Input: part model. Units: mm. Frame: model coordinates. Round coordinates to 2 decimals unless told otherwise and drop trailing zeros. Loops run counter-clockwise (first coordinate to the right, second up) from the corner with the lowest first, then second, coordinate; pieces in that order, holes last. Notation, with made-up numbers: (30.5, 13.5) - (75.5, 13.5) arc R5 cw to (75.5, 19.5) - close; hole circle Ø8 at (53, 24). An arc over 180 degrees is marked (long way). One line per question, with ' | ' between items. Start each with the question number.
Item 1: Section C-C, the plane z = -57. Return loops of the section in (x, y).
Item 2: Section B-B, the plane y = 1.5. Give the number of separate pieces and of enclosed holes in the cut face, plus the area to 3 significant figures.
Item 3: Section D-D, the plane x = -14. Return loops of the section in (y, z).
Item 4: First-contact query: pin 1 (0.6 mm diameter, centred on y = 1.5, z = -15.5, fed in from +X); pin 2 (12 mm diameter, centred on x = -7.5, z = -46.5, fed in from +Y). Flat tips, straight axial feed; report the tip coordinate or a pass-through.
Item 5: Material intervals for line 1 along Z through (x, y) = (-30, 1.25); line 2 along X through (y, z) = (1.2, -56); line 3 along Z through (x, y) = (-21.5, 0.7), sorted ascending.
Item 6: Section A-A, the plane x = -26. Return loops of the section in (y, z), plus the area to 3 significant figures.
Autodesk Inventor part; units mm, degrees
ref_plane "YZ Plane" through (0, 0, 0) normal (1, 0, 0) x (0, 1, 0)
ref_plane "XZ Plane" through (0, 0, 0) normal (0, 1, 0) x (-1, 0, 0)
ref_plane "XY Plane" through (0, 0, 0) normal (0, 0, 1) x (1, 0, 0)
sketch "Sketch1" plane through (0, 0, 0) normal (0, 1, 0) x (-1, 0, 0)
  line L0 (0, 0) -> (0, -30)
  line L1 (0, 0) -> (0.75, 0) construction
  arc A0 (1.4548, 0.2565) -> (0, 0) centre (0.75, 0) ccw
  line L2 (1.4548, 0.2565) -> (6.5322, -13.6936)
  line L3 (0, -30) -> (0.75, -30) construction
  circle A1 centre (0.75, -30) radius 0.75
  line L4 (1.0065, -30.7048) -> (6.5322, -28.6936)
  line L5 (6.5322, -13.6936) -> (6.5322, -28.6936) construction
  line L6 (6.5322, -13.6936) -> (35.2454, -42.4068)
  line L7 (6.5322, -13.6936) -> (66.5322, -13.6936) construction
  line L8 (6.5322, -28.6936) -> (27.7454, -49.9068)
  line L9 (6.5322, -28.6936) -> (36.5322, -28.6936) construction
  line L10 (27.7454, -49.9068) -> (27.7454, -58.9068)
  line L11 (27.7454, -58.9068) -> (6.5322, -80.12)
  line L12 (27.7454, -58.9068) -> (57.7454, -58.9068) construction
  line L13 (35.2454, -42.4068) -> (27.7454, -49.9068) construction
  arc A2 (36.7987, -46.1568) -> (35.2454, -42.4068) centre (31.4954, -46.1568) ccw
  line L14 (36.7987, -46.1568) -> (36.7987, -62.6568)
  line L15 (27.7454, -58.9068) -> (27.7454, -73.9068) construction
  line L16 (27.7454, -73.9068) -> (16.5322, -85.12)
  line L17 (27.7454, -73.9068) -> (35.2454, -66.4068)
  line L18 (27.7454, -58.9068) -> (35.2454, -66.4068) construction
  arc A3 (35.2454, -66.4068) -> (36.7987, -62.6568) centre (31.4954, -62.6568) ccw
  line L19 (6.5322, -80.12) -> (16.5322, -80.12) construction
  line L20 (16.5322, -80.12) -> (16.5322, -85.12) construction
  line L21 (16.5322, -110.12) -> (6.5322, -110.12)
  line L22 (6.5322, -110.12) -> (6.5322, -80.12)
  line L23 (16.5322, -85.12) -> (16.5322, -110.12)
  circle A4 centre (11.5322, -87.62) radius 2
  circle A5 centre (11.5322, -102.62) radius 2
  line L24 (0, -3.6658) -> (-2.5, -3.6658)
  line L25 (-2.5, -3.6658) -> (-2.5, -6.1658)
  line L26 (-2.5, -6.1658) -> (0, -6.1658)
  line L27 (0, -6.1658) -> (0, -3.6658)
  line L28 (-2.5, -3.6658) -> (0, -2.5)
  line L29 (-2.5, -6.1658) -> (0, -7.3315)
  line L30 (0, -10.9973) -> (-2.5, -10.9973)
  line L31 (-2.5, -10.9973) -> (-2.5, -13.4973)
  line L32 (-2.5, -13.4973) -> (0, -13.4973)
  line L33 (-2.5, -10.9973) -> (0, -9.8315)
  line L34 (-2.5, -13.4973) -> (0, -14.6631)
  line L35 (-2.5, -18.3288) -> (-2.5, -20.8288)
  line L36 (-2.5, -20.8288) -> (0, -21.9946)
  line L37 (-2.5, -20.8288) -> (0, -20.8288)
  line L38 (0, -18.3288) -> (-2.5, -18.3288)
  line L39 (-2.5, -18.3288) -> (0, -17.1631)
  line L40 (-2.5, -25.6604) -> (0, -24.4946)
  line L41 (0, -25.6604) -> (-2.5, -25.6604)
  line L42 (-2.5, -25.6604) -> (-2.5, -28.1604)
  line L43 (-2.5, -28.1604) -> (0, -28.1604)
  line L44 (-2.5, -28.1604) -> (0, -29.3262)
  circle A6 centre (6.5322, -21.1936) radius 2
  circle A7 centre (31.4954, -46.1568) radius 2
  circle A8 centre (31.4954, -62.6568) radius 2
  line L45 (18.0663, -78.6361) -> (18.0663, -68.0295)
  line L46 (20.5412, -81.111) -> (18.0663, -78.6361)
  line L47 (38.2189, -63.4333) -> (20.5412, -81.111)
  line L48 (38.2189, -63.4333) -> (30.4407, -55.6551)
  line L49 (18.0663, -68.0295) -> (30.4407, -55.6551)
  line L50 (18.0663, -78.6361) -> (18.0663, -83.5859)
  point P0 (18.0663, -68.5859)
  dimension "d2" = 30
  dimension "d17" = 0.75
  dimension "d18" = 20
  dimension "d19" = 0.75
  dimension "d20" = 70
  dimension "d21" = 15
  dimension "d28" = 45
  dimension "d29" = 30
  dimension "d30" = 45
  dimension "d31" = 9
  dimension "d34" = 135
  dimension "d35" = 15
  dimension "d36" = 135
  dimension "d38" = 10
  dimension "d39" = 30
  dimension "d40" = 30
  dimension "d41" = 7.5
  dimension "d42" = 5
  dimension "d43" = 7.5
  dimension "d44" = 5
  dimension "d45" = 4
  dimension "d46" = 4
  dimension "d47" = 2.5
  dimension "d48" = 2.5
  dimension "d49" = 25
  dimension "d50" = 25
  dimension "d51" = 2.5
  dimension "d52" = 2.5
  dimension "d53" = 2.5
  dimension "d54" = 25
  dimension "d55" = 25
  dimension "d56" = 2.5
  dimension "d57" = 2.5
  dimension "d58" = 2.5
  dimension "d59" = 25
  dimension "d60" = 25
  dimension "d61" = 2.5
  dimension "d62" = 2.5
  dimension "d63" = 2.5
  dimension "d64" = 25
  dimension "d65" = 25
  dimension "d66" = 2.5
  dimension "d69" = 4
  dimension "d70" = 4
  dimension "d71" = 4
extrude "Extrusion2" add sketch "Sketch1" along normal blind 2 contours A0 L2 L6 A2 L14 L48 L49 L10 L8 L4 A1 L0 | L0 L24 L28 | L0 L26 L25 L24 | L0 L29 L26 | L0 L30 L33 | L14 A3 L17 L16 L46 L45 L11 L10 L49 L48 | L0 L32 L31 L30 | L0 L34 L32 | L0 L38 L39 | L16 L50 L46 | L0 L37 L35 L38 | A1 | L0 L36 L37 | L44 L43 L0 | L0 L41 L40 | L43 L42 L41 L0
properties part number "claw_dynamic_gripper"
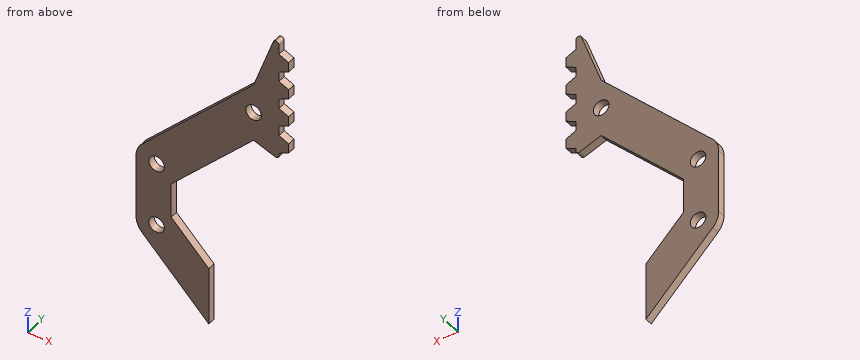
Return value:
1) outline: (-36.8, 0) - (-27.75, 0) - (-27.75, 2) - (-36.8, 2) - close
2) separate pieces: 1 | enclosed holes: 3 | area: 894 mm2
3) outline: (0, -36.16) - (2, -36.16) - (2, -21.16) - (0, -21.16) - close
4) pin 1: x = 0 | pin 2: through
5) line 1: -71.65 to -63.98, -61.33 to -47.48, -44.83 to -37.16 | line 2: -36.8 to -27.75 | line 3: -80.15 to -65.15, -43.66 to -28.66
6) outline: (0, -75.65) - (2, -75.65) - (2, -60.65) - (0, -60.65) - close; (0, -48.16) - (2, -48.16) - (2, -33.16) - (0, -33.16) - close | area: 60.0 mm2
